Check sheet for the modelled part. Datum: model origin and axes. Units: mm. A direction names the side the tool comes from. Round coordinates to 2 decimals unless told otherwise and drop trailing zeros. Write each loop counter-clockwise with the first axis right and the second up, starting at its lowest first coordinate (ties: lowest second). Pieces come first, ordered by that corner, then holes. Notation, with made-up numbers: (57, 19) -> (100, 19) arc R21 ccw to (100, 50) -> close; hole circle Ø8 at (-5.5, -20). An arc over 180 degrees is marked (long way). Write item = value, one per line.
from build123d import *

# Parameters (mm, degrees)
SKETCH1_W                  = 25
SKETCH1_H                  = 15
SKETCH2_R                  = 12.7
BOSS_EXTRUDE1_DEPTH        = 3
SKETCH3_R                  = 22.4917
BOSS_EXTRUDE2_DEPTH        = 65
F_10_CLEARANCE_HOLE1_D     = 5
F_10_CLEARANCE_HOLE1_DEPTH = 8
F_10_CLEARANCE_HOLE2_D     = 5
F_10_CLEARANCE_HOLE2_DEPTH = 12.446


with BuildPart() as part:
    # Sketch1 → Revolve1 (revolve)
    with BuildSketch(Plane.XZ):
        with Locations((12.5, 72.5)):
            Rectangle(SKETCH1_W, SKETCH1_H)
    revolve(axis=Axis((0, 0, 80), (0, 0, -1)))

    # Sketch2 → Boss-Extrude1 (add)
    with BuildSketch(Plane.XY.offset(80)):
        Circle(SKETCH2_R)
    extrude(amount=BOSS_EXTRUDE1_DEPTH)

    # Sketch3 → Boss-Extrude2 (add)
    with BuildSketch(Plane(origin=(0, 0, 65), x_dir=(-1, 0, 0), z_dir=(0, 0, -1))):
        Circle(SKETCH3_R)
    extrude(amount=BOSS_EXTRUDE2_DEPTH)

    # #10 Clearance Hole1
    with Locations(Plane(origin=(0, 0, 0), x_dir=(-1, 0, 0), z_dir=(0, 0, -1))):
        with Locations((-12.374368671, 12.374368671), (-17.5, 0), (-12.374368671, -12.374368671), (0, -17.5), (12.374368671, -12.374368671), (17.5, 0), (12.374368671, 12.374368671), (0, 17.5)):
            Hole(F_10_CLEARANCE_HOLE1_D / 2, depth=F_10_CLEARANCE_HOLE1_DEPTH)

    # #10 Clearance Hole2
    with Locations(Plane.XY.offset(80)):
        with Locations((-19.05, 0), (0, -19.05), (19.05, 0), (0, 19.05)):
            Hole(F_10_CLEARANCE_HOLE2_D / 2, depth=F_10_CLEARANCE_HOLE2_DEPTH)


solid = part.part
(1) Material ranges on L1, parallel to Y at x = 0, z = 71.25; L2, parallel to Y at x = 0, z = 4; L3, parallel to Z at x = -19.5, y = -2.5, recorded low to high. Write a range as [from, to].
Worked answers:
L1 = [-25, -21.55], [-16.55, 16.55], [21.55, 25]
L2 = [-22.49, -20], [-15, 15], [20, 22.49]
L3 = [0, 80]
(2) Release check for a two-part mould opening along X. For faces 4 (the flat face through (11.5, -5.9, 80)), 5 (the cylindrical face through (-2.75, -12.4, 81.48)), 6 (the cylindrical face through (-9.99, -11.62, 4.06)) record: pulls with the +X half, pulls with the -X half, needs draft (parallel to the pull), parting line crosses it, or undercut.
Worked answers:
face_4 = needs draft
face_5 = parting line crosses it
face_6 = undercut
(3) Go/stop test with flat-tipped pins: P1, Ø1.5, axis at x = 18, y = 1, coming from the +Z side; P2, Ø12, axis at x = -6, z = 56.5, coming from the +Y side; P3, Ø6, axis at x = 12.5, y = 5, coming from the -Z side; P4, Ø1.5, axis at x = 13.5, y = -12.5, coming from the -Z side. Record where each tip stops, or that it passes through.
Worked answers:
P1 = 67.55
P2 = 22.49
P3 = 0
P4 = 8
(4) Sectioned sample at C-C on z = 49. Enter the section's corners in (x, y).
Worked answers:
outline = circle Ø44.98 at (0, 0)
(5) Sectioned sample at A-A on x = 0. Enter the section's corners in (y, z).
Worked answers:
outline = (-25, 65) -> (-22.49, 65) -> (-22.49, 0) -> (-20, 0) -> (-20, 8) -> (-15, 8) -> (-15, 0) -> (15, 0) -> (15, 8) -> (20, 8) -> (20, 0) -> (22.49, 0) -> (22.49, 65) -> (25, 65) -> (25, 80) -> (21.55, 80) -> (21.55, 67.55) -> (16.55, 67.55) -> (16.55, 80) -> (12.7, 80) -> (12.7, 83) -> (-12.7, 83) -> (-12.7, 80) -> (-16.55, 80) -> (-16.55, 67.55) -> (-21.55, 67.55) -> (-21.55, 80) -> (-25, 80) -> close
(6) Sectioned sample at D-D on x = 19.05. Enter the section's corners in (y, z), then the cut area to 3 significant figures.
Worked answers:
outline = (-16.19, 65) -> (-11.96, 65) -> (-11.96, 0) -> (-1.96, 0) -> (-1.96, 8) -> (1.96, 8) -> (1.96, 0) -> (11.96, 0) -> (11.96, 65) -> (16.19, 65) -> (16.19, 80) -> (2.5, 80) -> (2.5, 67.55) -> (-2.5, 67.55) -> (-2.5, 80) -> (-16.19, 80) -> close
area = 1,950 mm²
(7) Sectioned sample at B-B on y = -9. Enter the section's corners in (x, z).
Worked answers:
outline = (-23.32, 65) -> (-20.61, 65) -> (-20.61, 0) -> (20.61, 0) -> (20.61, 65) -> (23.32, 65) -> (23.32, 80) -> (8.96, 80) -> (8.96, 83) -> (-8.96, 83) -> (-8.96, 80) -> (-23.32, 80) -> close
(8) Access from +Z, -Z, +X, -X, +Y, -Y to the whole of each face (thin tool, end or side, straight path). Record for faces 1 (the flat face through (0, 0, 83)), 2 (the flat face through (12, -12, 8)), 3 (the flat face through (-19, 0, 67.554)).
Worked answers:
face_1 = +Z, +X, -X, +Y, -Y
face_2 = -Z
face_3 = +Z
